```python
from build123d import *

# Parameters (mm, degrees)
ESQUISSE1_R      = 1.325
EXTRUSION1_DEPTH = 7.9
ESQUISSE2_R      = 1.75
EXTRUSION2_DEPTH = 2.1
ESQUISSE3_R      = 0.9
EXTRUSION3_DEPTH = 3
ESQUISSE4_R      = 1.15
EXTRUSION4_DEPTH = 2.1
CONG_1_R         = 1.15
CHANFREIN1_SIZE  = 0.2
CHANFREIN1_SIZE2 = 0.346410162


with BuildPart() as part:
    # Esquisse1 → Extrusion1 (new body)
    with BuildSketch(Plane.XY):
        Circle(ESQUISSE1_R)
    extrude(amount=EXTRUSION1_DEPTH)

    # Esquisse2 → Extrusion2 (add)
    with BuildSketch(Plane.XY.offset(7.9)):
        Circle(ESQUISSE2_R)
    extrude(amount=EXTRUSION2_DEPTH)

    # Esquisse3 → Extrusion3 (add)
    with BuildSketch(Plane.XY.offset(10)):
        Circle(ESQUISSE3_R)
    extrude(amount=EXTRUSION3_DEPTH)

    # Esquisse4 → Extrusion4 (add)
    with BuildSketch(Plane.XY.offset(13)):
        Circle(ESQUISSE4_R)
    extrude(amount=EXTRUSION4_DEPTH)

    # Congé1
    cong_1_edges = [part.edges().sort_by_distance(p)[0] for p in [
        (-1.15, 0, 15.1),
    ]]
    fillet(cong_1_edges, radius=CONG_1_R)

    # Chanfrein1
    chanfrein1_edges = [part.edges().sort_by_distance(p)[0] for p in [
        (-1.75, 0, 10),
    ]]
    chanfrein1_side = [part.faces().sort_by_distance(p)[0] for p in [
        (-1.700502525, 0, 10),
    ]]
    chamfer(chanfrein1_edges, length=CHANFREIN1_SIZE, length2=CHANFREIN1_SIZE2, reference=chanfrein1_side[0])


solid = part.part
```
CAD build for the part. Positions are in the model's coordinates, mm. A direction names the side the tool comes from. Coordinates: 2 decimals unless noted, no trailing zeros. Write each loop counter-clockwise with the first axis right and the second up, starting at its lowest first coordinate (ties: lowest second). Pieces come first, ordered by that corner, then holes.
(1) 3-axis set-ups, long thin cutter, end or side, ignore diameter. For faces 1 (the face through (1.617, -0.67, 8.765)), 2 (the face through (-0.91, -0.7, 13.47)): which of +Z, -Z, +X, -X, +Y, -Y reach the whole face in a straight line?
(2) Cut at C-C, the plane z = 7. List the corners of the cut face in (x, y) (3 decimals), and give its area (3 significant figures).
(3) Drill centre lines: probe 1 along X at (y, z) = (-0.1, 8.5); probe 2 along Z at (x, y) = (1.15, -0.4); probe 3 along Z at (x, y) = (-0.05, 1.45). Where is each one in solid material? Low to high.
(4) Two-plate mould, pull along Z, no slides. Class faces 3 (the face through (0.32, -1.01, 10)), 4 (the face through (1.224, -0.507, 3.895)), 5 (the face through (0, 0, 0)), 6 (the face through (0.86, 0.27, 11.48)): +Z half, -Z half, draft (parallel to the pull), parting line (faces both ways), or undercut.
(5) Flat gauge pins, fed straight in: pin 1 (1.5 mm diameter, centred on x = 0.5, z = 13.5, fed in from +Y); pin 2 (1.5 mm diameter, centred on y = -0.5, z = 6, fed in from -X) (3 decimals). Where does each tip first touch, or does it go through?
(6) Cut at A-A, the plane y = 0. List the corners of the cut face in (x, z) (3 decimals), and give its area (3 significant figures).
Geometry says:
1. face 1: +Z, -Z
1. face 2: +Z
2. outline: circle Ø2.65 at (0, 0)
2. area: 5.52 mm2
3. probe 1: x = -1.75 to 1.75
3. probe 2: z = 0 to 10
3. probe 3: z = 7.9 to 10
4. face 3: undercut
4. face 4: draft
4. face 5: -Z half
4. face 6: undercut
5. pin 1: stops at y = 1.15
5. pin 2: stops at x = -1.325
6. outline: (-1.75, 7.9) - (-1.325, 7.9) - (-1.325, 0) - (1.325, 0) - (1.325, 7.9) - (1.75, 7.9) - (1.75, 9.654) - (1.55, 10) - (0.9, 10) - (0.9, 13) - (1.15, 13) - (1.15, 13.95) arc R1.15 ccw to (-1.15, 13.95) - (-1.15, 13) - (-0.9, 13) - (-0.9, 10) - (-1.55, 10) - (-1.75, 9.654) - close
6. area: 37.9 mm2
